Geometry: final body of the model. Coordinates: model frame, mm. Face numbers are marked on the shaded views. A direction names the side the tool comes from. Round coordinates to 2 decimals unless told otherwise and drop trailing zeros. Write each loop counter-clockwise with the first axis right and the second up, starting at its lowest first coordinate (ties: lowest second). Pieces come first, ordered by that corner, then holes. Notation, with made-up numbers: M 46,-4.75 L 70,-4.75 A16 cw 70,10.25 Z; hole C -8,31 d10. An arc over 180 degrees is marked long. Use one line per item in the form item = value. Start each with the question number.
from build123d import *

# Parameters (mm, degrees)
F0_W     = 69.961674
F0_H     = 68.511577
F1_DEPTH = 40.132
F2_W     = 32.101594
F2_H     = 36.901384
F3_DEPTH = 85.852
F4_R     = 5.08


with BuildPart() as f1:
    # F0 (on Top) → F1 (new body)
    with BuildSketch(Plane.XY):
        with Locations((5.486086, -11.040198)):
            Rectangle(F0_W, F0_H)
    extrude(amount=F1_DEPTH)

    # F2 (on Front) → F3 (join)
    with BuildSketch(Plane.XZ):
        with Locations((1.719728, 28.49517)):
            Rectangle(F2_W, F2_H)
    extrude(amount=F3_DEPTH)

    # F4
    f4_edges = [f1.edges().sort_by_distance(p)[0] for p in [
        (17.770525, -42.926, 46.945862),
        (-14.331069, -42.926, 46.945862),
        (1.719728, 0, 46.945862),
        (1.719728, -85.852, 46.945862),
    ]]
    fillet(f4_edges, radius=F4_R)


solid = f1.part
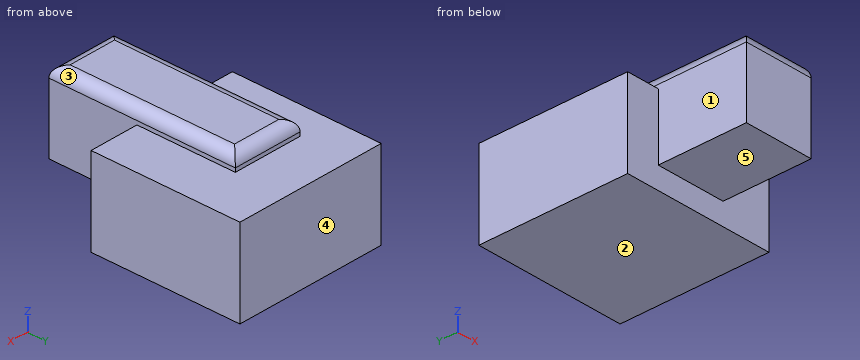
1. Section query C-C (y = -6.5). Return loops of the section in (x, z).
2. Ray query, probe 1 along Y at (x, z) = (-17, 8.5); probe 2 along X at (y, z) = (-51.5, 22); probe 3 along Z at (x, y) = (0, 0.5). Return the intervals inside material, ascending.
3. Contact query for flat-ended pins moving along their axis: pin 1 (0.5 mm diameter, centred on x = 7, z = 41, fed in from +Y); pin 2 (6 mm diameter, centred on x = 32, z = 14.5, fed in from -Y). Output: stop coordinate, or through.
4. Pull-direction query (Z, two-part tool) for the marked faces 1, 2 and 3; classes: released by +Z, released by -Z, zero draft, split by the parting line, or undercut.
5. Set-up query: the marked faces 4 and 5. Return all of +Z, -Z, +X, -X, +Y, -Y with unobstructed straight access to the full face (end or side cutting, diameter ignored); none if empty.
6. Section query D-D (y = -54). Return loops of the section in (x, z).
7. Section query A-A (x = -4.5). Return loops of the section in (y, z).
8. Section query B-B (z = 21). Return loops of the section in (x, y).
Checks:
q1.outline = M -29.49,0 L 40.47,0 L 40.47,40.13 L 17.77,40.13 L 17.77,41.87 A5.08 ccw 12.69,46.95 L -9.25,46.95 A5.08 ccw -14.33,41.87 L -14.33,40.13 L -29.49,40.13 Z
q2.probe_1 = -45.3 to 23.22
q2.probe_2 = -14.33 to 17.77
q2.probe_3 = 0 to 40.13
q3.pin_1 = 0
q3.pin_2 = -45.3
q4.face_1 = zero draft
q4.face_2 = released by -Z
q4.face_3 = released by +Z
q5.face_4 = +Z, -Z, +X, -X, +Y
q5.face_5 = -Z, +X, -X, -Y
q6.outline = M -14.33,10.04 L 17.77,10.04 L 17.77,41.87 A5.08 ccw 12.69,46.95 L -9.25,46.95 A5.08 ccw -14.33,41.87 Z
q7.outline = M -85.85,10.04 L -45.3,10.04 L -45.3,0 L 23.22,0 L 23.22,40.13 L 0,40.13 L 0,41.87 A5.08 ccw -5.08,46.95 L -80.77,46.95 A5.08 ccw -85.85,41.87 Z
q8.outline = M -29.49,-45.3 L -14.33,-45.3 L -14.33,-85.85 L 17.77,-85.85 L 17.77,-45.3 L 40.47,-45.3 L 40.47,23.22 L -29.49,23.22 Z
